The drawing under review shows one solid part. Ordinate dimensions are in mm from its lowest x, y, z. A direction names the side the tool comes from. Give positions to 0.01 mm unless a question says otherwise; leave off trailing zeros. Loops run counter-clockwise (first coordinate to the right, second up) from the corner with the lowest first, then second, coordinate; pieces in that order, holes last.
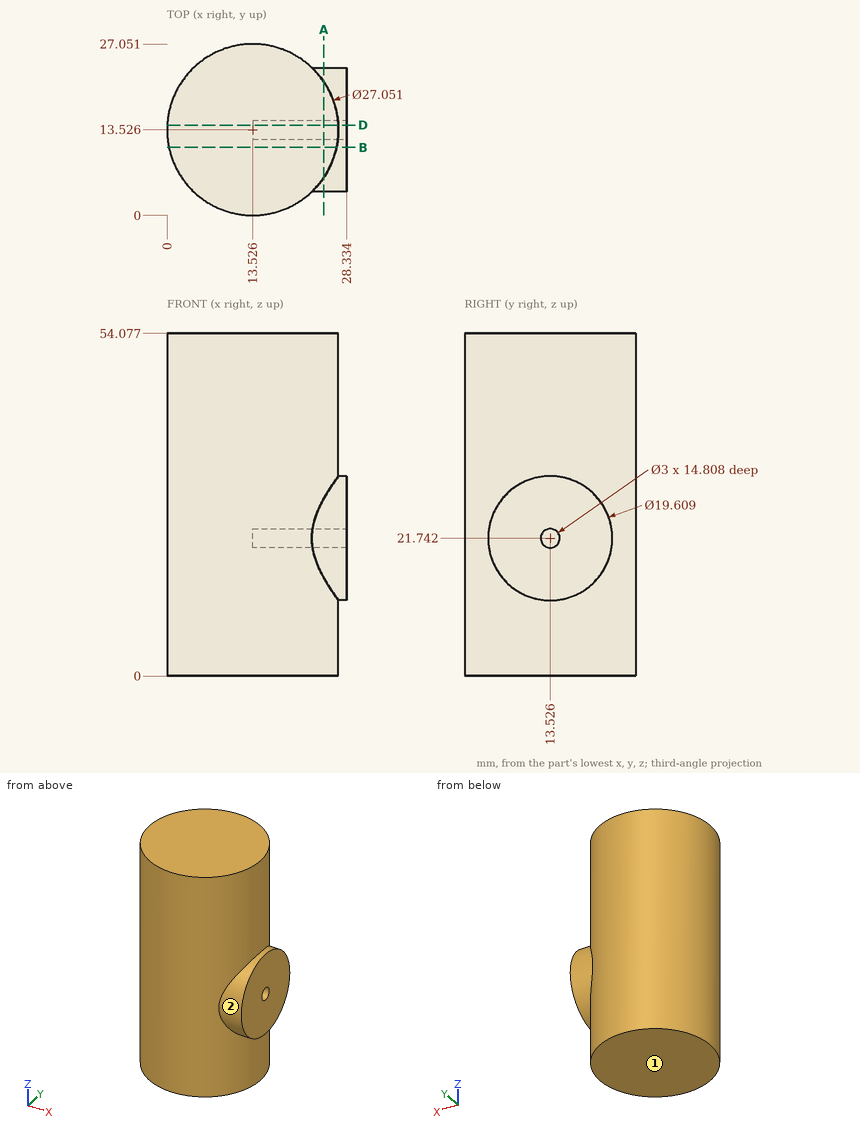
Item 1: Take a section at A-A on x = 24.75. Give the boundary of the cut face in (y, z) (1 decimal), and give its area (3 significant figures).
Answer:
outline: (6, 0) - (21.1, 0) - (21.1, 15.5) arc R9.8 ccw to (21.1, 28) - (21.1, 54.1) - (6, 54.1) - (6, 28) arc R9.8 ccw to (6, 15.5) - close; hole circle Ø3 at (13.5, 21.7)
area: 848 mm2
Item 2: Tool access review of the marked faces 1 and 2: name each direction out of +Z, -Z, +X, -X, +Y, -Y from which nothing blocks a thin tool from reaching the whole face with its end or side.
Answer:
face 1: -Z, +X, -X, +Y, -Y
face 2: +X
Item 3: Clearance check with flat-ended pins moving along their axes: pin 1 Ø4 at (y, z) = (17.5, 7) entering from +X; pin 2 Ø4 at (x, z) = (19, 21.5) entering from -Y; pin 3 Ø2 at (x, z) = (21, 18.5) entering from -Y. State where each tip first meets the part, or that it passes through.
Answer:
pin 1: stops at x = 26.91
pin 2: stops at y = 0.45
pin 3: stops at y = 1.65
Item 4: Take a section at B-B on y = 10.75. Give the boundary of the cut face in (x, z) (1 decimal), and give its area (3 significant figures).
Answer:
outline: (0.3, 0) - (26.8, 0) - (26.8, 12.3) - (28.3, 12.3) - (28.3, 31.1) - (26.8, 31.1) - (26.8, 54.1) - (0.3, 54.1) - close
area: 1,460 mm2
Item 5: Take a section at D-D on y = 14.25. Give the boundary of the cut face in (x, z) (1 decimal).
Answer:
outline: (0, 0) - (27, 0) - (27, 12) - (28.3, 12) - (28.3, 20.4) - (13.5, 20.4) - (13.5, 23.1) - (28.3, 23.1) - (28.3, 31.5) - (27, 31.5) - (27, 54.1) - (0, 54.1) - close
Item 6: For L1, parallel to Y at x = 17.75, z = 22 (1 decimal); L2, parallel to Y at x = 25.25, z = 12 (1 decimal); L3, parallel to X at y = 21.5, z = 4.5, list the stretches that pass through material, from the lowest coordinate up.
Answer:
L1: y = 0.7 to 12, 15 to 26.4
L2: y = 6.8 to 20.3
L3: x = 2.6 to 24.45
